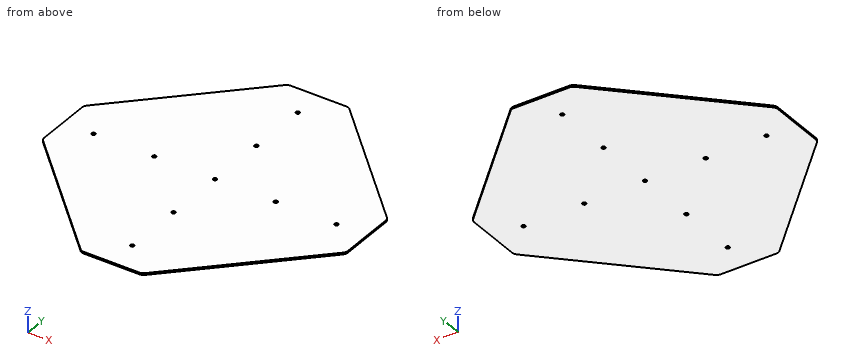
```python
from build123d import *

# Parameters (mm, degrees)
SKETCH1_R           = 1.651
BOSS_EXTRUDE1_DEPTH = 1.5875


with BuildPart() as part:
    # Sketch1 → Boss-Extrude1 (new body)
    with BuildSketch(Plane(origin=(0, 0, 0), x_dir=(-1, 0, 0), z_dir=(0, 0, -1))):
        with BuildLine():
            Line((-133.310112052, -28.614887943), (-28.614887941, -133.310112054))
            ThreePointArc((-28.614887941, -133.310112054), (-26.812310708, -134.514555654), (-24.686025887, -134.937500002))
            Line((-24.686025887, -134.937500002), (24.68602589, -134.937500002))
            ThreePointArc((24.68602589, -134.937500002), (26.812310711, -134.514555654), (28.614887944, -133.310112054))
            Line((28.614887944, -133.310112054), (133.310112056, -28.614887942))
            ThreePointArc((133.310112056, -28.614887942), (134.514555656, -26.81231071), (134.937500003, -24.686025888))
            Line((134.937500003, -24.686025888), (134.937500003, 24.686025887))
            ThreePointArc((134.937500003, 24.686025887), (134.514555656, 26.812310709), (133.310112056, 28.614887942))
            Line((133.310112056, 28.614887942), (28.614887944, 133.310112054))
            ThreePointArc((28.614887944, 133.310112054), (26.812310711, 134.514555654), (24.68602589, 134.937500001))
            Line((24.68602589, 134.937500001), (-24.686025886, 134.937500001))
            ThreePointArc((-24.686025886, 134.937500001), (-26.812310708, 134.514555654), (-28.614887941, 133.310112054))
            Line((-28.614887941, 133.310112054), (-133.310112053, 28.614887942))
            ThreePointArc((-133.310112053, 28.614887942), (-134.514555652, 26.81231071), (-134.9375, 24.686025888))
            Line((-134.9375, 24.686025888), (-134.9375, -24.686025888))
            ThreePointArc((-134.9375, -24.686025888), (-134.514555652, -26.81231071), (-133.310112052, -28.614887943))
        make_face()
        with Locations((0, 53.975)):
            Circle(SKETCH1_R, mode=Mode.SUBTRACT)
        Circle(SKETCH1_R, mode=Mode.SUBTRACT)
        with Locations((0, -107.95)):
            Circle(SKETCH1_R, mode=Mode.SUBTRACT)
        with Locations((0, 107.95)):
            Circle(SKETCH1_R, mode=Mode.SUBTRACT)
        with Locations((-53.975, 0)):
            Circle(SKETCH1_R, mode=Mode.SUBTRACT)
        with Locations((53.975, 0)):
            Circle(SKETCH1_R, mode=Mode.SUBTRACT)
        with Locations((0, -53.975)):
            Circle(SKETCH1_R, mode=Mode.SUBTRACT)
        with Locations((-107.95, 0)):
            Circle(SKETCH1_R, mode=Mode.SUBTRACT)
        with Locations((107.95, 0)):
            Circle(SKETCH1_R, mode=Mode.SUBTRACT)
    extrude(amount=-BOSS_EXTRUDE1_DEPTH)


solid = part.part
```
Model file for the job. Use its own axes, mm. Give positions to 0.01 mm unless a question says otherwise; leave off trailing zeros. Write each loop counter-clockwise with the first axis right and the second up, starting at its lowest first coordinate (ties: lowest second). Pieces come first, ordered by that corner, then holes. Notation, with made-up numbers: (-38.75, -7.75) - (-10.75, -7.75) arc R14 ccw to (-10.75, -0.75) - close; hole circle Ø7 at (-29.75, 12). An arc over 180 degrees is marked (long way). One line per question, with ' | ' between items. Start each with the question number.
(1) Slice it at A-A on z = 1.15. Give the number of separate pieces and of enclosed holes in the cut face, plus the area to 3 significant figures.
(2) Slice it at C-C on x = 35.5. Write the cut outline in (y, z) (1 decimal).
(3) Wall check: line 1 along Y through (x, z) = (0, 0.55); line 2 along Y through (x, z) = (-0.5, 1.1); line 3 along X through (y, z) = (-44.5, 1.05) (3 decimals). Give the ranges that are in metal, low to high. Write a range as from..to.
(4) Slice it at B-B on y = 95. Write the cut outline in (x, z) (1 decimal), plus the area to 3 significant figures.
Results below:
1) separate pieces: 1 | enclosed holes: 9 | area: 49,400 mm^2
2) outline: (-126.4, 0) - (126.4, 0) - (126.4, 1.6) - (-126.4, 1.6) - close
3) line 1: -134.94..-109.6, -106.3..-55.63, -52.32..-1.65, 1.65..52.32, 55.63..106.3, 109.6..134.94 | line 2: -134.94..-109.52, -106.38..-55.55, -52.4..-1.57, 1.57..52.4, 55.55..106.38, 109.52..134.94 | line 3: -117.425..117.425
4) outline: (-66.9, 0) - (66.9, 0) - (66.9, 1.6) - (-66.9, 1.6) - close | area: 212 mm^2
